Design review of the part built by this model. Coordinates are the model's own, in mm. Face numbers are marked on the shaded views. A direction names the side the tool comes from. Round coordinates to 2 decimals unless told otherwise and drop trailing zeros. Write each loop counter-clockwise with the first axis right and the second up, starting at its lowest first coordinate (ties: lowest second). Pieces come first, ordered by that corner, then holes. Notation, with made-up numbers: (43.5, 81) - (86.5, 81) arc R20 cw to (86.5, 88) - close; hole circle Ø1 at (-18, 35.5). An arc over 180 degrees is marked (long way). Use one line per item in the form item = value.
```python
from build123d import *

# Parameters (mm, degrees)
F0_W     = 49.427262
F0_H     = 20
F1_DEPTH = 10
F2_W     = 10.004918
F2_H     = 2.53289
F3_DEPTH = 9
F4_R     = 7
F5_R     = 1.254098
F6_DEPTH = 10.001


with BuildPart() as f1:
    # F0 (on Top) → F1 (new body)
    with BuildSketch(Plane.XY):
        Rectangle(F0_W, F0_H)
    extrude(amount=F1_DEPTH)

    # F2 (on face) → F3 (cut)
    with BuildSketch(Plane.XY.offset(10)):
        with Locations((-15.424379, 3.665117)):
            Rectangle(F2_W, F2_H)
        with BuildLine():
            Line((-10.42192, 0.878937), (-12.701521, 0.878937))
            Line((-12.701521, 0.878937), (-12.701521, 0.245714))
            ThreePointArc((-12.701521, 0.245714), (-12.678233, -0.099326), (-12.701521, -0.444367))
            ThreePointArc((-12.701521, -0.444367), (-13.552341, -2.029358), (-15.234413, -2.66711))
            Line((-15.234413, -2.66711), (-20.553483, -2.66711))
            Line((-20.553483, -2.66711), (-20.553483, -5.2))
            Line((-20.553483, -5.2), (-13.717022, -5.2))
            ThreePointArc((-13.717022, -5.2), (-11.387862, -4.235716), (-10.42192, -1.907243))
            Line((-10.42192, -1.907243), (-10.42192, 0.878937))
        make_face()
        with BuildLine():
            ThreePointArc((-12.701521, -0.444367), (-12.678233, -0.099326), (-12.701521, 0.245714))
            Line((-12.701521, 0.245714), (-12.701521, -0.444367))
        make_face()
        with BuildLine():
            Line((-6.369294, 4.931562), (-9.155474, 4.931562))
            Line((-9.155474, 4.931562), (-9.155474, -4.693422))
            ThreePointArc((-9.155474, -4.693422), (-7.228804, -3.922643), (-6.369294, -2.033887))
            Line((-6.369294, -2.033887), (-6.369294, 4.931562))
        make_face()
        with BuildLine():
            Line((-0.037068, 4.931562), (-2.696603, 4.931562))
            Line((-2.696603, 4.931562), (-2.696603, -1.907243))
            ThreePointArc((-2.696603, -1.907243), (-2.679752, -2.097209), (-2.696603, -2.287176))
            ThreePointArc((-2.696603, -2.287176), (-2.882546, -2.726977), (-3.24005, -3.043506))
            ThreePointArc((-3.24005, -3.043506), (-3.759009, -3.176466), (-4.277969, -3.043506))
            Line((-4.277969, -3.043506), (-5.329138, -3.043506))
            ThreePointArc((-5.329138, -3.043506), (-5.889298, -4.314902), (-6.960199, -5.2))
            Line((-6.960199, -5.2), (-6.369294, -5.2))
            Line((-6.369294, -5.2), (-2.443314, -5.2))
            ThreePointArc((-2.443314, -5.2), (-0.805329, -4.703243), (-0.037068, -3.173688))
            Line((-0.037068, -3.173688), (-0.037068, 4.931562))
        make_face()
        with BuildLine():
            ThreePointArc((-2.696603, -2.287176), (-2.679752, -2.097209), (-2.696603, -1.907243))
            Line((-2.696603, -1.907243), (-2.696603, -2.287176))
        make_face()
        with BuildLine():
            ThreePointArc((-4.277969, -3.043506), (-3.759009, -3.176466), (-3.24005, -3.043506))
            Line((-3.24005, -3.043506), (-4.277969, -3.043506))
        make_face()
        with BuildLine():
            Line((4.09889, 4.95471), (1.31271, 4.95471))
            Line((1.31271, 4.95471), (1.31271, 2.398672))
            Line((1.31271, 2.398672), (1.31271, -4.670274))
            ThreePointArc((1.31271, -4.670274), (3.23938, -3.899495), (4.09889, -2.010739))
            Line((4.09889, -2.010739), (4.09889, 2.398672))
            Line((4.09889, 2.398672), (7.771581, 2.398672))
            Line((7.771581, 2.398672), (7.771581, -1.884095))
            ThreePointArc((7.771581, -1.884095), (7.788432, -2.074061), (7.771581, -2.264028))
            ThreePointArc((7.771581, -2.264028), (7.585638, -2.703829), (7.228134, -3.020358))
            ThreePointArc((7.228134, -3.020358), (6.709175, -3.153318), (6.190215, -3.020358))
            Line((6.190215, -3.020358), (5.139046, -3.020358))
            ThreePointArc((5.139046, -3.020358), (4.578886, -4.291754), (3.507985, -5.176852))
            Line((3.507985, -5.176852), (4.09889, -5.176852))
            Line((4.09889, -5.176852), (8.02487, -5.176852))
            ThreePointArc((8.02487, -5.176852), (9.662855, -4.680095), (10.431116, -3.15054))
            Line((10.431116, -3.15054), (10.431116, 2.398672))
            Line((10.431116, 2.398672), (10.431116, 4.95471))
            Line((10.431116, 4.95471), (7.771581, 4.95471))
            Line((7.771581, 4.95471), (4.09889, 4.95471))
        make_face()
        with BuildLine():
            ThreePointArc((7.771581, -2.264028), (7.788432, -2.074061), (7.771581, -1.884095))
            Line((7.771581, -1.884095), (7.771581, -2.264028))
        make_face()
        with BuildLine():
            ThreePointArc((6.190215, -3.020358), (6.709175, -3.153318), (7.228134, -3.020358))
            Line((7.228134, -3.020358), (6.190215, -3.020358))
        make_face()
        with BuildLine():
            Line((14.5961, 5.087933), (11.809921, 5.087933))
            Line((11.809921, 5.087933), (11.809921, -4.537051))
            ThreePointArc((11.809921, -4.537051), (13.73659, -3.766272), (14.5961, -1.877516))
            Line((14.5961, -1.877516), (14.5961, 5.087933))
        make_face()
        with BuildLine():
            Line((20.928327, 5.087933), (18.268792, 5.087933))
            Line((18.268792, 5.087933), (18.268792, -1.750871))
            ThreePointArc((18.268792, -1.750871), (18.285642, -1.940838), (18.268792, -2.130805))
            ThreePointArc((18.268792, -2.130805), (18.082849, -2.570606), (17.725345, -2.887134))
            ThreePointArc((17.725345, -2.887134), (17.206385, -3.020095), (16.687426, -2.887134))
            Line((16.687426, -2.887134), (15.636256, -2.887134))
            ThreePointArc((15.636256, -2.887134), (15.076097, -4.158531), (14.005196, -5.043629))
            Line((14.005196, -5.043629), (14.5961, -5.043629))
            Line((14.5961, -5.043629), (18.522081, -5.043629))
            ThreePointArc((18.522081, -5.043629), (20.160066, -4.546872), (20.928327, -3.017317))
            Line((20.928327, -3.017317), (20.928327, 5.087933))
        make_face()
        with BuildLine():
            ThreePointArc((18.268792, -2.130805), (18.285642, -1.940838), (18.268792, -1.750871))
            Line((18.268792, -1.750871), (18.268792, -2.130805))
        make_face()
        with BuildLine():
            ThreePointArc((16.687426, -2.887134), (17.206385, -3.020095), (17.725345, -2.887134))
            Line((17.725345, -2.887134), (16.687426, -2.887134))
        make_face()
    extrude(amount=-F3_DEPTH, mode=Mode.SUBTRACT)

    # F4
    f4_edges = [f1.edges().sort_by_distance(p)[0] for p in [
        (-24.713631, 10, 5),
        (24.713631, -10, 5),
    ]]
    fillet(f4_edges, radius=F4_R)

    # F5 (on face) → F6 (cut, through all)
    with BuildSketch(Plane.XY.offset(10)):
        with Locations((22.113672, 7.445175)):
            Circle(F5_R)
    extrude(amount=-F6_DEPTH, mode=Mode.SUBTRACT)


solid = f1.part
```
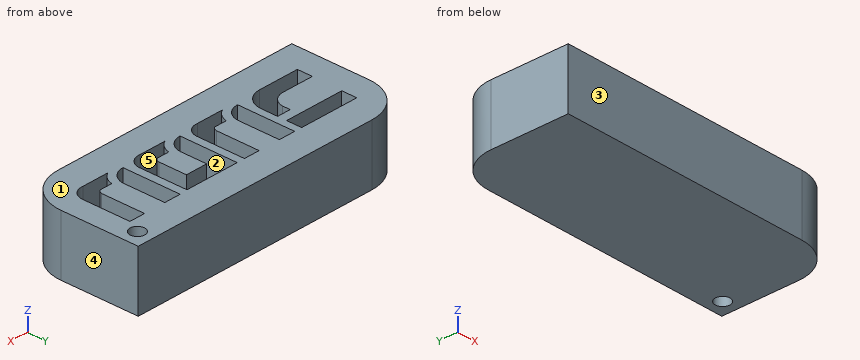
Q1. Draft analysis for pull direction Y (two halves, no side actions). For the marked faces 3, 4 and 5, state which applies: released by +Y, released by -Y, zero draft, split by the parting line, or undercut.
Calculated:
face_3 = released by -Y
face_4 = zero draft
face_5 = undercut
Q2. Machinability: for the marked faces 1 and 2, which of the approach directions +Z, -Z, +X, -X, +Y, -Y give a long, thin tool a straight path to every point of the face, cutting with its end or side? Answer none if there is none.
Calculated:
face_1 = +Z, +X, -X, +Y, -Y
face_2 = +Z
Q3. To check wall thickness, follow line 1 along Y through (x, z) = (-2.5, 3.25); line 2 along Y through (x, z) = (-16.5, 5); line 3 along Y through (x, z) = (18, 2). State the ranges of each line that lie inside material, in increasing order. Write a range as from..to.
Calculated:
line_1 = -10..-5.2, 4.93..10
line_2 = -10..-5.2, -2.67..2.4, 4.93..10
line_3 = -9.99..-5.04, -2.67..10
Q4. We need section D-D on x = 20. Write out the cut boundary in (y, z).
Calculated:
outline = (-9.62, 0) - (10, 0) - (10, 10) - (5.09, 10) - (5.09, 1) - (-4.67, 1) - (-4.67, 10) - (-9.62, 10) - close
Q5. For P1, Ø1.3, axis at x = 19, z = 4, coming from the -Y side; P2, Ø1.5, axis at x = 13, y = 1, coming from the +Z side, all flat-tipped, find the tip position at first contact; note any pin that passes through.
Calculated:
P1 = -9.97
P2 = 1
Q6. We need section C-C on z = 5.5. State how many separate pieces and enclosed holes the cut face has, then the cut area to 3 significant figures.
Calculated:
separate_pieces = 1
enclosed_holes = 8
area = 721 mm2
Q7. We need section B-B on x = -2. Write out the cut boundary in (y, z).
Calculated:
outline = (-10, 0) - (10, 0) - (10, 10) - (4.93, 10) - (4.93, 1) - (-5.2, 1) - (-5.2, 10) - (-10, 10) - close
